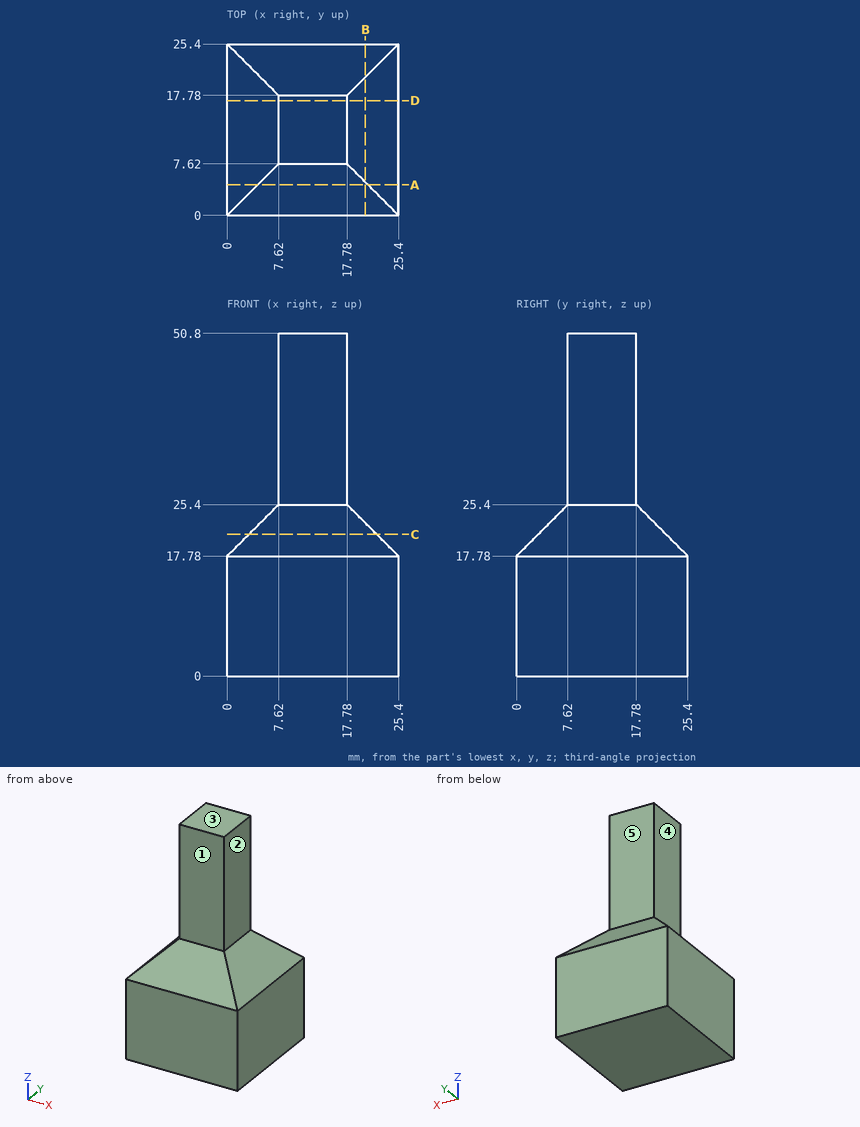
The drawing under review shows one solid part. Ordinate dimensions are in mm from its lowest x, y, z. A direction names the side the tool comes from. Give positions to 0.01 mm unless a question says otherwise; leave off trailing zeros. Write each loop counter-clockwise with the first axis right and the second up, starting at its lowest first coordinate (ties: lowest second). Pieces come first, ordered by that corner, then holes. Notation, with made-up numbers: (-3.5, -39) -> (53.5, -39) arc R17 cw to (53.5, -31) -> close; hole circle Ø3 at (28.5, -4.75). An arc over 180 degrees is marked (long way). Use CSV: the item, a comma, the result in double quotes.
Q1. For P1, Ø5, axis at x = 13.5, z = 39, coming from the -Y side; P2, Ø8, axis at y = 11.5, z = 40.5, coming from the -X side; P3, Ø2, axis at x = 14.5, z = 24, coming from the -Y side; P4, Ø3, axis at x = 14.5, y = 19.5, coming from the -Z side, all flat-tipped, find the tip position at first contact; note any pin that passes through.
Conclusion:
P1,"y = 7.62"
P2,"x = 7.62"
P3,"y = 5.22"
P4,"z = 0"
Q2. To check wall thickness, follow probe 1 along Y at (x, z) = (12, 47.5); probe 2 along Z at (x, y) = (16.5, 4.5); probe 3 along Z at (x, y) = (16.5, 4). State the ranges of each line that lie inside material, in increasing order. Write a range as [from, to].
Conclusion:
probe 1,"[7.62, 17.78]"
probe 2,"[0, 22.28]"
probe 3,"[0, 21.78]"
Q3. Take a section at C-C, the plane z = 21. Write out the cut boundary in (x, y), then the cut area to 3 significant figures.
Conclusion:
outline,"(3.22, 3.22) -> (22.18, 3.22) -> (22.18, 22.18) -> (3.22, 22.18) -> close"
area,"359 mm2"
Q4. Take a section at B-B, the plane x = 20.5. Write out the cut boundary in (y, z), then the cut area to 3 significant figures.
Conclusion:
outline,"(0, 0) -> (25.4, 0) -> (25.4, 17.78) -> (20.5, 22.68) -> (4.9, 22.68) -> (0, 17.78) -> close"
area,"552 mm2"
Q5. Tool access review of the marked faces 1, 2, 3, 4 and 5: name each direction out of +Z, -Z, +X, -X, +Y, -Y from which nothing blocks a thin tool from reaching the whole face with its end or side.
Conclusion:
face 1,"+Z, +X, -X, -Y"
face 2,"+Z, +X, +Y, -Y"
face 3,"+Z, +X, -X, +Y, -Y"
face 4,"+Z, -X, +Y, -Y"
face 5,"+Z, +X, -X, +Y"
Q6. Take a section at D-D, the plane y = 17. Write out the cut boundary in (x, z), then the cut area to 3 significant figures.
Conclusion:
outline,"(0, 0) -> (25.4, 0) -> (25.4, 17.78) -> (17.78, 25.4) -> (17.78, 50.8) -> (7.62, 50.8) -> (7.62, 25.4) -> (0, 17.78) -> close"
area,"845 mm2"
Q7. Take a section at A-A, the plane y = 4.5. Write out the cut boundary in (x, z).
Conclusion:
outline,"(0, 0) -> (25.4, 0) -> (25.4, 17.78) -> (20.9, 22.28) -> (4.5, 22.28) -> (0, 17.78) -> close"
